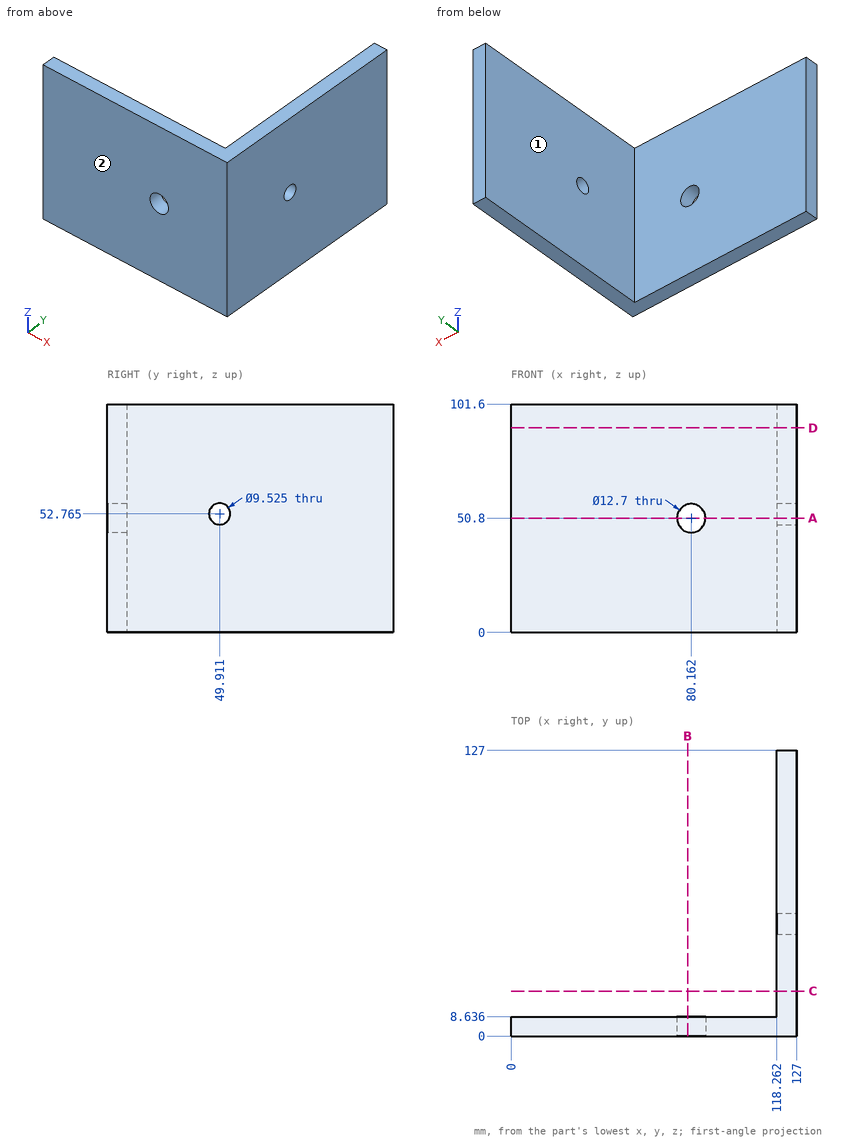
Answer from the drawing. Dimensions are ordinates in mm from the lowest x, y and z of the part. A direction names the side the tool comes from. Round coordinates to 2 decimals unless told otherwise and drop trailing zeros. Loops run counter-clockwise (first coordinate to the right, second up) from the corner with the lowest first, then second, coordinate; pieces in that order, holes last.
(1) The part is cut by section D-D, the plane z = 91. Give the vertices of the cut face in (x, y), and give its area (3 significant figures).
Computed values:
outline: (0, 0) - (127, 0) - (127, 127) - (118.26, 127) - (118.26, 8.64) - (0, 8.64) - close
area: 2,130 mm2
(2) The part is cut by section A-A, the plane z = 50.8. Give the vertices of the cut face in (x, y), and give its area (3 significant figures).
Computed values:
outline: (0, 0) - (73.81, 0) - (73.81, 8.64) - (0, 8.64) - close; (86.51, 0) - (127, 0) - (127, 45.57) - (118.26, 45.57) - (118.26, 8.64) - (86.51, 8.64) - close; (118.26, 54.25) - (127, 54.25) - (127, 127) - (118.26, 127) - close
area: 1,950 mm2
(3) The part is cut by section C-C, the plane y = 20. Give the vertices of the cut face in (x, z).
Computed values:
outline: (118.26, 0) - (127, 0) - (127, 101.6) - (118.26, 101.6) - close
(4) Each of these flat-tipped pins is pushed along its axis until it touches: P1, Ø16.5, axis at x = 80.16, z = 50.8, coming from the +Y side; P2, Ø10, axis at y = 75, z = 71, coming from the -X side. Where does it stop, or does it pass through?
Computed values:
P1: stops at y = 8.64
P2: stops at x = 118.26
(5) The part is cut by section B-B, the plane x = 78.5. Give the vertices of the cut face in (y, z).
Computed values:
outline: (0, 0) - (8.64, 0) - (8.64, 44.67) - (0, 44.67) - close; (0, 56.93) - (8.64, 56.93) - (8.64, 101.6) - (0, 101.6) - close
(6) For the marked faces 1 and 2, determine the directions among +Z, -Z, +X, -X, +Y, -Y from which every point of the face is accessible in a straight line to the end or side of a thin tool.
Computed values:
face 1: +Z, -Z, -X, +Y
face 2: +Z, -Z, +X, -X, -Y
(7) Find the intervals of material crossed by L1, parallel to Y at x = 109.5, z = 78; L2, parallel to X at y = 98, z = 54, in increasing order.
Computed values:
L1: y = 0 to 8.64
L2: x = 118.26 to 127
